Model file for the job. Use its own axes, mm. Round coordinates to 2 decimals unless told otherwise and drop trailing zeros. Loops run counter-clockwise (first coordinate to the right, second up) from the corner with the lowest first, then second, coordinate; pieces in that order, holes last. Notation, with made-up numbers: M 17,23 L 62,23 A33 cw 62,55 Z; hole C -25.75,78.5 d10. An arc over 180 degrees is marked long. Use a Markdown table: item, result. Add a question column.
Q1. Cut at C-C (x = 25). Give the cut face in (y, z), plus the area to 3 significant figures.
Q2. Cut at A-A (x = -3.5). Give the cut face in (y, z).
Q3. Probe line 1 (Y direction, x = 36, z = 3.8); line 2 (X direction, y = -29.5, z = 1.45); line 3 (X direction, y = -33, z = 4.75). List the from-to ranges inside material, lowest first. Write a range as from..to.
Q4. Pin check, flat tips, straight feed: pin 1 (6 mm diameter, centred on x = -5.5, y = -42.5, fed in from +Z); pin 2 (1 mm diameter, centred on y = 40.5, z = 4, fed in from -X). Stop position of each tip, or through.
Q5. Cut at B-B (x = -23.5). Give the cut face in (y, z).
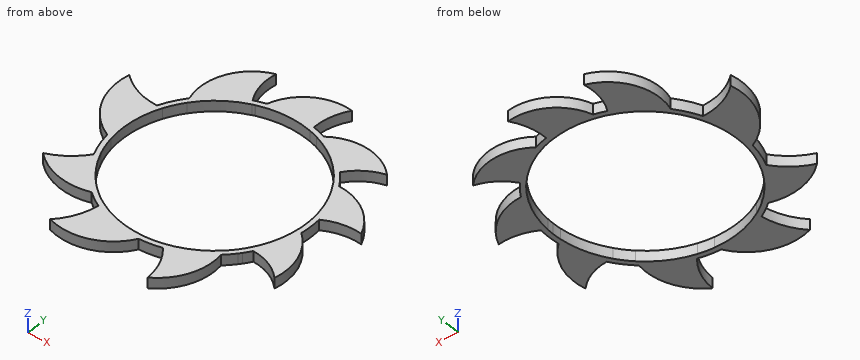
from build123d import *

# Parameters (mm, degrees)
F1_DEPTH = 5


with BuildPart() as f1:
    # F0 (on Top) → F1 (new body)
    with BuildSketch(Plane.XY):
        with BuildLine():
            ThreePointArc((38.502261, -1.597772), (40.718756, 0.748882), (43.205982, 2.806393))
            ThreePointArc((43.205982, 2.806393), (41.074175, 13.694702), (36.245186, 23.683733))
            ThreePointArc((36.245186, 23.683733), (34.607614, 26.018181), (32.819931, 28.239774))
            ThreePointArc((32.819931, 28.239774), (24.499086, 35.699124), (14.546237, 40.780383))
            ThreePointArc((14.546237, 40.780383), (12.950133, 39.127779), (11.519659, 37.329894))
            ThreePointArc((11.519659, 37.329894), (10.939992, 39.638686), (10.562187, 41.988961))
            ThreePointArc((10.562187, 41.988961), (-1.797083, 43.259718), (-14.008372, 40.968258))
            ThreePointArc((-14.008372, 40.968258), (-14.033128, 40.846587), (-14.058419, 40.725026))
            ThreePointArc((-14.058419, 40.725026), (-14.150281, 40.80644), (-14.242495, 40.887456))
            ThreePointArc((-14.242495, 40.887456), (-14.802375, 40.688111), (-15.359467, 40.4811))
            ThreePointArc((-15.359467, 40.4811), (-25.8155, 34.759065), (-34.315088, 26.402792))
            ThreePointArc((-34.315088, 26.402792), (-36.969234, 22.536824), (-39.189715, 18.40649))
            ThreePointArc((-39.189715, 18.40649), (-42.897454, 5.868657), (-42.693446, -7.20433))
            ThreePointArc((-42.693446, -7.20433), (-41.725569, -11.558959), (-40.314768, -15.790888))
            ThreePointArc((-40.314768, -15.790888), (-34.506812, -26.151723), (-26.101976, -34.544457))
            ThreePointArc((-26.101976, -34.544457), (-23.851243, -33.463072), (-21.70451, -32.187641))
            ThreePointArc((-21.70451, -32.187641), (-21.539561, -34.851521), (-21.608116, -37.519622))
            ThreePointArc((-21.608116, -37.519622), (-9.843426, -42.16325), (2.76125, -43.20889))
            ThreePointArc((2.76125, -43.20889), (3.776863, -40.777994), (4.55104, -38.259785))
            ThreePointArc((4.55104, -38.259785), (7.293587, -40.055986), (9.795652, -42.174375))
            ThreePointArc((9.795652, -42.174375), (20.620392, -38.071408), (29.97107, -31.246882))
            ThreePointArc((29.97107, -31.246882), (29.244852, -28.952192), (28.314719, -26.732316))
            ThreePointArc((28.314719, -26.732316), (31.777465, -25.55893), (35.383111, -24.953319))
            ThreePointArc((35.383111, -24.953319), (40.599644, -15.043325), (43.099902, -4.126874))
            ThreePointArc((43.099902, -4.126874), (40.863438, -2.748966), (38.502261, -1.597772))
        make_face()
        with BuildLine():
            ThreePointArc((11.090625, 36.944765), (11.091742, 36.830639), (11.092309, 36.716508))
            ThreePointArc((11.092309, 36.716508), (11.076055, 36.692352), (11.059829, 36.668176))
            ThreePointArc((11.059829, 36.668176), (11.075017, 36.806494), (11.090625, 36.944765))
        make_face(mode=Mode.SUBTRACT)
        with BuildLine():
            add(Edge.make_bspline(
                [(35.924434, -28.145118), (35.55734, -28.595677), (35.190245, -29.046235), (34.82315, -29.496794)],
                knots=[0, 0, 0, 0, 1.743518, 1.743518, 1.743518, 1.743518], degree=3))
            ThreePointArc((35.924434, -28.145118), (37.12508, -26.541309), (38.254179, -24.88635))
            ThreePointArc((38.254179, -24.88635), (42.839633, -15.731451), (45.268646, -5.784669))
            ThreePointArc((45.268646, -5.784669), (45.630344, -0.76446), (45.437012, 4.265048))
            ThreePointArc((45.437012, 4.265048), (43.311152, 14.382515), (38.962614, 23.761888))
            ThreePointArc((38.962614, 23.761888), (36.690962, 27.138275), (34.127567, 30.298875))
            ThreePointArc((34.127567, 30.298875), (26.090127, 37.44353), (16.603983, 42.509063))
            ThreePointArc((16.603983, 42.509063), (13.529918, 43.58502), (10.386943, 44.438993))
            ThreePointArc((10.386943, 44.438993), (-0.500898, 45.633998), (-11.359886, 44.20029))
            ThreePointArc((-11.359886, 44.20029), (-14.046385, 43.421328), (-16.680117, 42.479246))
            ThreePointArc((-16.680117, 42.479246), (-26.848804, 36.903311), (-35.283704, 28.944307))
            ThreePointArc((-35.283704, 28.944307), (-38.912407, 23.844019), (-41.809082, 18.295172))
            ThreePointArc((-41.809082, 18.295172), (-45.198145, 6.31192), (-45.22164, -6.141333))
            ThreePointArc((-45.22164, -6.141333), (-43.969857, -12.221472), (-41.904528, -18.075485))
            ThreePointArc((-41.904528, -18.075485), (-36.350911, -27.592099), (-28.678272, -35.500273))
            ThreePointArc((-28.678272, -35.500273), (-25.385911, -37.924506), (-21.889795, -40.044345))
            ThreePointArc((-21.889795, -40.044345), (-10.586101, -44.391971), (1.46312, -45.613287))
            ThreePointArc((1.46312, -45.613287), (6.593302, -45.157956), (11.639511, -44.12748))
            ThreePointArc((11.639511, -44.12748), (21.699379, -40.147847), (30.539846, -33.912099))
            ThreePointArc((30.539846, -33.912099), (32.755977, -31.776699), (34.82315, -29.496794))
        make_face()
        with BuildLine():
            ThreePointArc((43.205982, 2.806393), (43.274261, 1.403935), (43.297029, 0))
            ThreePointArc((43.297029, 0), (43.247719, -2.06579), (43.099902, -4.126874))
            ThreePointArc((43.099902, -4.126874), (40.599644, -15.043325), (35.383111, -24.953319))
            ThreePointArc((35.383111, -24.953319), (32.828257, -28.230094), (29.97107, -31.246882))
            ThreePointArc((29.97107, -31.246882), (20.620392, -38.071408), (9.795652, -42.174375))
            ThreePointArc((9.795652, -42.174375), (6.299722, -42.836272), (2.76125, -43.20889))
            ThreePointArc((2.76125, -43.20889), (-9.843426, -42.16325), (-21.608116, -37.519622))
            ThreePointArc((-21.608116, -37.519622), (-23.901383, -36.10203), (-26.101976, -34.544457))
            ThreePointArc((-26.101976, -34.544457), (-34.506812, -26.151723), (-40.314768, -15.790888))
            ThreePointArc((-40.314768, -15.790888), (-41.725569, -11.558959), (-42.693446, -7.20433))
            ThreePointArc((-42.693446, -7.20433), (-42.897454, 5.868657), (-39.189715, 18.40649))
            ThreePointArc((-39.189715, 18.40649), (-36.969234, 22.536824), (-34.315088, 26.402792))
            ThreePointArc((-34.315088, 26.402792), (-25.8155, 34.759065), (-15.359467, 40.4811))
            ThreePointArc((-15.359467, 40.4811), (-14.802375, 40.688111), (-14.242495, 40.887456))
            ThreePointArc((-14.242495, 40.887456), (-14.125491, 40.928024), (-14.008372, 40.968258))
            ThreePointArc((-14.008372, 40.968258), (-1.797083, 43.259718), (10.562187, 41.988961))
            ThreePointArc((10.562187, 41.988961), (12.568747, 41.432587), (14.546237, 40.780383))
            ThreePointArc((14.546237, 40.780383), (24.499086, 35.699124), (32.819931, 28.239774))
            ThreePointArc((32.819931, 28.239774), (34.607614, 26.018181), (36.245186, 23.683733))
            ThreePointArc((36.245186, 23.683733), (41.074175, 13.694702), (43.205982, 2.806393))
        make_face(mode=Mode.SUBTRACT)
        with BuildLine():
            ThreePointArc((45.268646, -5.784669), (42.839633, -15.731451), (38.254179, -24.88635))
            ThreePointArc((38.254179, -24.88635), (46.836585, -26.9326), (54.002321, -32.080128))
            ThreePointArc((54.002321, -32.080128), (53.318598, -17.709102), (45.268646, -5.784669))
        make_face()
        with BuildLine():
            ThreePointArc((18.030986, -60.946237), (28.411333, -49.338255), (30.539846, -33.912099))
            ThreePointArc((30.539846, -33.912099), (21.699379, -40.147847), (11.639511, -44.12748))
            ThreePointArc((11.639511, -44.12748), (16.292682, -51.983004), (18.030986, -60.946237))
        make_face()
        with BuildLine():
            ThreePointArc((38.962614, 23.761888), (43.311152, 14.382515), (45.437012, 4.265048))
            ThreePointArc((45.437012, 4.265048), (53.655325, 7.364285), (62.435822, 7.585189))
            ThreePointArc((62.435822, 7.585189), (53.112392, 19.175175), (38.962614, 23.761888))
        make_face()
        with BuildLine():
            ThreePointArc((-30.59298, -57.094834), (-12.530174, -57.035031), (1.46312, -45.613287))
            ThreePointArc((1.46312, -45.613287), (-10.586101, -44.391971), (-21.889795, -40.044345))
            ThreePointArc((-21.889795, -40.044345), (-24.869098, -49.270056), (-30.59298, -57.094834))
        make_face()
        with BuildLine():
            ThreePointArc((16.603983, 42.509063), (26.090127, 37.44353), (34.127567, 30.298875))
            ThreePointArc((34.127567, 30.298875), (40.342926, 36.373929), (48.304058, 39.860666))
            ThreePointArc((48.304058, 39.860666), (32.956953, 47.204731), (16.603983, 42.509063))
        make_face()
        with BuildLine():
            ThreePointArc((-56.653903, -29.111429), (-43.535146, -36.111304), (-28.678272, -35.500273))
            ThreePointArc((-28.678272, -35.500273), (-36.350911, -27.592099), (-41.904528, -18.075485))
            ThreePointArc((-41.904528, -18.075485), (-48.504761, -24.628504), (-56.653903, -29.111429))
        make_face()
        with BuildLine():
            ThreePointArc((-11.359886, 44.20029), (-0.500898, 45.633998), (10.386943, 44.438993))
            ThreePointArc((10.386943, 44.438993), (11.475998, 52.869411), (15.087919, 60.564346))
            ThreePointArc((15.087919, 60.564346), (-1.180367, 57.302692), (-11.359886, 44.20029))
        make_face()
        with BuildLine():
            ThreePointArc((-60.702262, 25.645594), (-58.506458, 7.051887), (-45.22164, -6.141333))
            ThreePointArc((-45.22164, -6.141333), (-45.198145, 6.31192), (-41.809082, 18.295172))
            ThreePointArc((-41.809082, 18.295172), (-51.937891, 20.216839), (-60.702262, 25.645594))
        make_face()
        with BuildLine():
            ThreePointArc((-35.283704, 28.944307), (-26.848804, 36.903311), (-16.680117, 42.479246))
            ThreePointArc((-16.680117, 42.479246), (-19.699815, 50.753822), (-19.535904, 59.560655))
            ThreePointArc((-19.535904, 59.560655), (-33.732866, 47.504807), (-35.283704, 28.944307))
        make_face()
    extrude(amount=F1_DEPTH)


solid = f1.part
Checked values:
| question | item | result |
|---|---|---|
| 1 | outline | M -54.84,0 L -35.35,0 L -35.35,5 L -54.84,5 Z; M 35.35,0 L 46.53,0 L 46.53,5 L 35.35,5 Z |
| 1 | area | 153 mm^2 |
| 2 | outline | M -51.62,0 L -43.16,0 L -43.16,5 L -51.62,5 Z; M 43.16,0 L 55.67,0 L 55.67,5 L 43.16,5 Z |
| 3 | line 1 | y = -28.05..-24.05, 24.05..28.05, 32.62..46.75 |
| 3 | line 2 | x = -56.23..-31.69, 31.69..34.82, 51.14..54.46 |
| 3 | line 3 | x = -51.44..-28.03, 28.03..31.52 |
| 4 | pin 1 | stops at z = 5 |
| 4 | pin 2 | stops at x = -36.16 |
| 5 | outline | M -58.55,0 L -46.17,0 L -46.17,5 L -58.55,5 Z; M -39.12,0 L -36.36,0 L -36.36,5 L -39.12,5 Z; M 36.36,0 L 57.88,0 L 57.88,5 L 36.36,5 Z |
